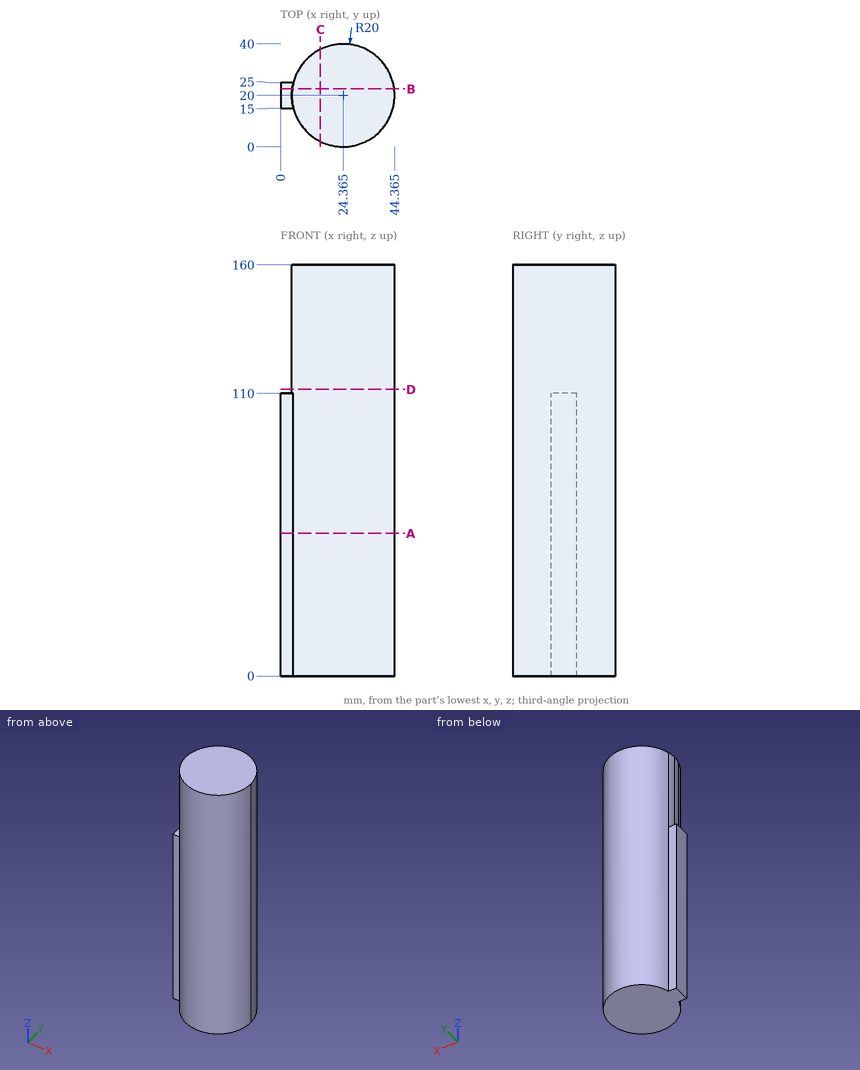
Job drawing, mm, ordinate dimensions from the low corner. One solid piece. Give positions to 0.01 mm unless a question says otherwise; leave off trailing zeros. Loops run counter-clockwise (first coordinate to the right, second up) from the corner with the lowest first, then second, coordinate; pieces in that order, holes last. Notation, with made-up numbers: (81, 62.25) -> (99, 62.25) arc R11 ccw to (99, 82.25) -> close; hole circle Ø9 at (47.25, 36). An arc over 180 degrees is marked (long way). Write each question's results on one line, items separated by ' | '. Start each with the question number.
Q1. Band-saw the part on C-C on x = 15.5. List the corners of the cut face in (y, z), plus the area to 3 significant figures.
Q2. Band-saw the part on B-B on y = 22.5. List the corners of the cut face in (x, z), plus the area to 3 significant figures.
Q3. Wall check: L1, parallel to Y at x = 19.5, z = 91.5; L2, parallel to Y at x = 27, z = 54; L3, parallel to X at y = 24.5, z = 63.5. Give the ranges that are in metal, low to high.
Q4. Band-saw the part on D-D on z = 111.5. List the corners of the cut face in (x, y) (3 decimals), plus the area to 3 significant figures.
Q5. Pin check, flat tips, straight feed: P1, Ø1.5, axis at x = 39.5, z = 143.5, coming from the +Y side (3 decimals); P2, Ø12, axis at x = 7.5, z = 97, coming from the -Y side; P3, Ø2.5, axis at x = 3, z = 67.5, coming from the +Y side. Stop position of each tip, or through.
Q6. Band-saw the part on A-A on z = 55.5. List the corners of the cut face in (x, y) (3 decimals).
Results are:
1) outline: (2.07, 0) -> (37.93, 0) -> (37.93, 160) -> (2.07, 160) -> close | area: 5,740 mm²
2) outline: (0, 0) -> (44.21, 0) -> (44.21, 160) -> (4.52, 160) -> (4.52, 110) -> (0, 110) -> close | area: 6,850 mm²
3) L1: y = 0.6 to 39.4 | L2: y = 0.17 to 39.83 | L3: x = 0 to 43.85
4) outline: circle Ø40 at (24.365, 20) | area: 1,260 mm²
5) P1: stops at y = 33.895 | P2: stops at y = 3.21 | P3: stops at y = 25
6) outline: (0, 15) -> (5, 15) arc R20 ccw (long way) to (5, 25) -> (0, 25) -> close
